For this review, take the finished solid that the model builds, in its own axes (mm). Coordinates: 2 decimals unless noted, no trailing zeros. Write each loop counter-clockwise with the first axis right and the second up, starting at its lowest first coordinate (ties: lowest second). Pieces come first, ordered by that corner, then holes.
1) We need section B-B on x = -38.5. Write out the cut boundary in (y, z), then the cut area to 3 significant figures.
2) We need section A-A on y = 312.5. Write out the cut boundary in (x, z) (3 decimals).
3) We need section C-C on y = 353. Give the number of separate pieces and of enclosed holes in the cut face, then the cut area to 3 significant figures.
4) To check wall thickness, follow line 1 along X through (y, z) = (323.5, 4) (3 decimals); line 2 along X through (y, z) = (338, 2) (3 decimals); line 3 along X through (y, z) = (343, 2) (3 decimals). State the ranges of each line that lie inside material, in increasing order.
5) Insertion check: P1, Ø8, axis at x = -16.5, y = 298, coming from the -Z side; P2, Ø1.9, axis at y = 340.5, z = 4.5, coming from the +X side; P3, Ø2, axis at x = 9, z = 3, coming from the -Y side; P4, Ø1.9, axis at y = 301, z = 1.5, coming from the +X side. Each pin has a flat end and moves straight along its axis. Give the tip position at first contact, or say it passes through.
from build123d import *

# Parameters (mm, degrees)
BOSS_EXTRUDE1_DEPTH = 6.35


with BuildPart() as part:
    # Sketch1 → Boss-Extrude1 (new body)
    with BuildSketch(Plane.XY):
        with BuildLine():
            Line((-53.175, 406.4), (-41.275, 406.4))
            Line((-41.275, 406.4), (-41.275, 412.75))
            Line((-41.275, 412.75), (-28.575, 412.75))
            Line((-28.575, 412.75), (-28.575, 406.4))
            Line((-28.575, 406.4), (-6.35, 406.4))
            Line((-6.35, 406.4), (22.225, 406.4))
            Line((22.225, 406.4), (22.225, 412.75))
            Line((22.225, 412.75), (34.925, 412.75))
            Line((34.925, 412.75), (34.925, 406.4))
            Line((34.925, 406.4), (46.825, 406.4))
            add(Edge.make_bspline(
                [(46.825, 406.4), (48.444514788, 362.591265004), (34.925, 323.85)],
                knots=[0, 0, 0, 0.535068669, 0.535068669, 0.535068669], degree=2))
            Line((34.925, 323.85), (34.925, 368.3))
            Line((34.925, 368.3), (28.575, 368.3))
            Line((28.575, 368.3), (28.575, 307.792730185))
            add(Edge.make_bspline(
                [(28.575, 307.792730185), (17.572742264, 282.971699721), (0, 260.35)],
                knots=[0.647499935, 0.647499935, 0.647499935, 1, 1, 1], degree=2))
            Line((0, 260.35), (0, 330.2))
            Line((0, 330.2), (-6.35, 330.2))
            Line((-6.35, 330.2), (-6.35, 260.35))
            add(Edge.make_bspline(
                [(-34.925, 307.792730185), (-23.922742264, 282.971699721), (-6.35, 260.35)],
                knots=[0.647499935, 0.647499935, 0.647499935, 1, 1, 1], degree=2))
            Line((-34.925, 307.792730185), (-34.925, 368.3))
            Line((-34.925, 368.3), (-41.275, 368.3))
            Line((-41.275, 368.3), (-41.275, 323.85))
            add(Edge.make_bspline(
                [(-53.175, 406.4), (-54.794514788, 362.591265004), (-41.275, 323.85)],
                knots=[0, 0, 0, 0.535068669, 0.535068669, 0.535068669], degree=2))
        make_face()
    extrude(amount=BOSS_EXTRUDE1_DEPTH)


solid = part.part
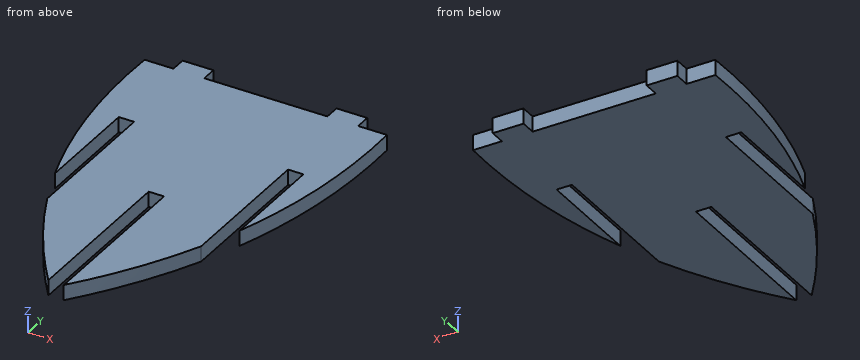
Result:
1. outline: (368.3, 0) - (412.75, 0) - (412.75, 6.35) - (368.3, 6.35) - close
1. area: 282 mm2
2. outline: (-34.925, 0) - (-6.35, 0) - (-6.35, 6.35) - (-34.925, 6.35) - close; (0, 0) - (28.575, 0) - (28.575, 6.35) - (0, 6.35) - close
3. separate pieces: 3
3. enclosed holes: 0
3. area: 503 mm2
4. line 1: x = -34.925 to -6.35, 0 to 28.575
4. line 2: x = -45.662 to -41.275, -34.925 to 28.575, 34.925 to 39.312
4. line 3: x = -46.957 to -41.275, -34.925 to 28.575, 34.925 to 40.607
5. P1: stops at z = 0
5. P2: stops at x = 40.22
5. P3: stops at y = 271.25
5. P4: stops at x = 25.88
